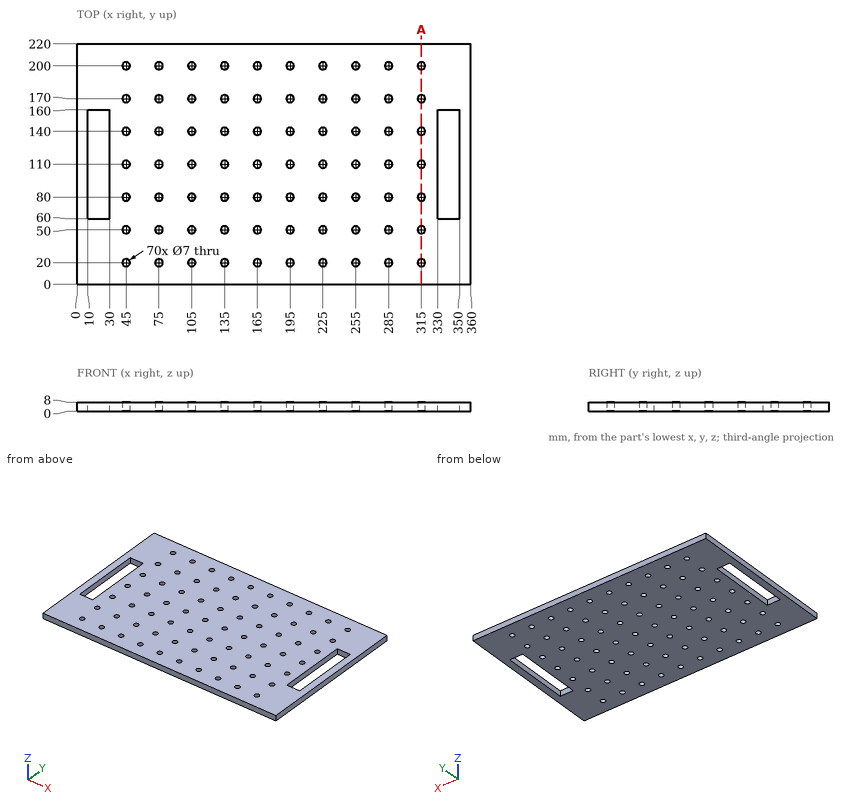
The drawing under review shows one solid part. Ordinate dimensions are in mm from its lowest x, y, z. Coordinates: 2 decimals unless noted, no trailing zeros. Put each result on its own line as item: value.
1) Wall thickness on probe 1 along X at (y, z) = (155.5, 7.25); probe 2 along Y at (x, z) = (15, 3.25): over which ranges is each line inside the solid? List them lowest first. Write a range as [from, to].
Computed:
probe 1: x = [0, 10], [30, 330], [350, 360]
probe 2: y = [0, 60], [160, 220]
2) Add section A-A on x = 315. State how many separate pieces and enclosed holes the cut face has, then the cut area to 3 significant figures.
Computed:
separate pieces: 8
enclosed holes: 0
area: 1,370 mm2
3) Clearance check with a flat-ended pin moving along its axis: pin 1 Ø4 at (x, y) = (135, 200) entering from -Z. State where the tip first meets the part, or that it passes through.
Computed:
pin 1: passes through
